Verification items for the finished model (mm, model axes). A direction names the side the tool comes from. Give positions to 0.01 mm unless a question says otherwise; leave off trailing zeros. Write each loop counter-clockwise with the first axis right and the second up, starting at its lowest first coordinate (ties: lowest second). Pieces come first, ordered by that corner, then holes. Notation, with made-up numbers: M 9,50.25 L 40,50.25 A9 ccw 40,62.25 Z; hole C 17,-22.75 d1. An arc over 180 degrees is marked long. Write item = value, one per line.
from build123d import *

# Parameters (mm, degrees)
SKETCH1_W           = 68.58
SKETCH1_H           = 26.67
SKETCH1_W_2         = 63.5
SKETCH1_H_2         = 5
BOSS_EXTRUDE1_DEPTH = 3.175
FILLET1_R           = 1.27


with BuildPart() as part:
    # Sketch1 → Boss-Extrude1 (new body)
    with BuildSketch(Plane.XY):
        Rectangle(SKETCH1_W, SKETCH1_H)
        Polygon((-20.750635985, 10.795), (0, 2.725308228), (20.750635985, 10.795), align=None, mode=Mode.SUBTRACT)
        with Locations((0, -7.025)):
            Rectangle(SKETCH1_W_2, SKETCH1_H_2, mode=Mode.SUBTRACT)
        Polygon((-31.75, 9.621913994), (-31.75, -1.985), (-7.007935444, 0), align=None, mode=Mode.SUBTRACT)
        Polygon((7.007935444, 0), (31.75, 9.621913994), (31.75, -1.985), align=None, mode=Mode.SUBTRACT)
    extrude(amount=BOSS_EXTRUDE1_DEPTH)

    # Fillet1
    fillet1_edges = [part.edges().sort_by_distance(p)[0] for p in [
        (20.750635985, 10.795, 1.5875),
        (-20.750635985, 10.795, 1.5875),
        (0, 2.725308228, 1.5875),
        (-7.007935444, 0, 1.5875),
        (-31.75, 9.621913994, 1.5875),
        (-31.75, -1.985, 1.5875),
        (7.007935444, 0, 1.5875),
        (31.75, -1.985, 1.5875),
        (31.75, 9.621913994, 1.5875),
    ]]
    fillet(fillet1_edges, radius=FILLET1_R)


solid = part.part
1) Cross-section at A-A on y = -6. Record the boundary of the cut face in (x, z) (3 decimals).
From the geometry:
outline = M -34.29,0 L -31.75,0 L -31.75,3.175 L -34.29,3.175 Z; M 31.75,0 L 34.29,0 L 34.29,3.175 L 31.75,3.175 Z
2) Draft check along X on faces 1 (the flat face through (0, -13.335, 2)), 2 (the flat face through (34.29, 0, 2)), 3 (the flat face through (0, 10.795, 2)). Enter one of: +X half, -X half, draft (parallel to the pull), parting line (faces both ways), or undercut.
From the geometry:
face_1 = draft
face_2 = +X half
face_3 = undercut
3) Cross-section at C-C on x = -5. Record the boundary of the cut face in (y, z) (3 decimals), plus the area to 3 significant figures.
From the geometry:
outline = M -13.335,0 L -9.525,0 L -9.525,3.175 L -13.335,3.175 Z; M -4.525,0 L 4.67,0 L 4.67,3.175 L -4.525,3.175 Z; M 10.795,0 L 13.335,0 L 13.335,3.175 L 10.795,3.175 Z
area = 49.4 mm^2
4) Cross-section at D-D on x = -21.5. Record the boundary of the cut face in (y, z) (3 decimals).
From the geometry:
outline = M -13.335,0 L -9.525,0 L -9.525,3.175 L -13.335,3.175 Z; M -4.525,0 L -1.163,0 L -1.163,3.175 L -4.525,3.175 Z; M 5.636,0 L 13.335,0 L 13.335,3.175 L 5.636,3.175 Z
5) Material ranges on probe 1 along X at (y, z) = (1, 0.85); probe 2 along Y at (x, z) = (-0.5, 1.95) (3 decimals); probe 3 along Y at (x, z) = (13.5, 1.4) (3 decimals), recorded low to high. Write a range as from..to.
From the geometry:
probe_1 = -34.29..-31.75, -11.37..11.37, 31.75..34.29
probe_2 = -13.335..-9.525, -4.525..2.92, 10.795..13.335
probe_3 = -13.335..-9.525, -4.525..-0.521, 2.525..7.975, 10.795..13.335
6) Tool access check on faces 4 (the flat face through (0, 13.335, 2)), 5 (the flat face through (21.58, -1.17, 1.57)). Record the directions out of +Z, -Z, +X, -X, +Y, -Y that give a thin tool (end or side, any length) a straight path to the whole face; none if there is none.
From the geometry:
face_4 = +Z, -Z, +X, -X, +Y
face_5 = +Z, -Z
7) Cross-section at B-B on z = 2.6. Record the boundary of the cut face in (x, y) (3 decimals), plus the area to 3 significant figures.
From the geometry:
outline = M -34.29,-13.335 L 34.29,-13.335 L 34.29,13.335 L -34.29,13.335 Z; hole M -31.75,-9.525 L 31.75,-9.525 L 31.75,-4.525 L -31.75,-4.525 Z; hole M -31.75,-0.609 A1.27 ccw -30.378,-1.875 L -12.527,-0.443 A1.27 ccw -12.168,2.007 L -30.02,8.949 A1.27 ccw -31.75,7.765 Z; hole M -14.441,8.341 L -0.46,2.904 A1.27 ccw 0.46,2.904 L 14.441,8.341 A1.27 ccw 13.981,10.795 L -13.981,10.795 A1.27 ccw Z; hole M 12.168,2.007 A1.27 ccw 12.527,-0.443 L 30.378,-1.875 A1.27 ccw 31.75,-0.609 L 31.75,7.765 A1.27 ccw 30.02,8.949 Z
area = 1,080 mm^2
